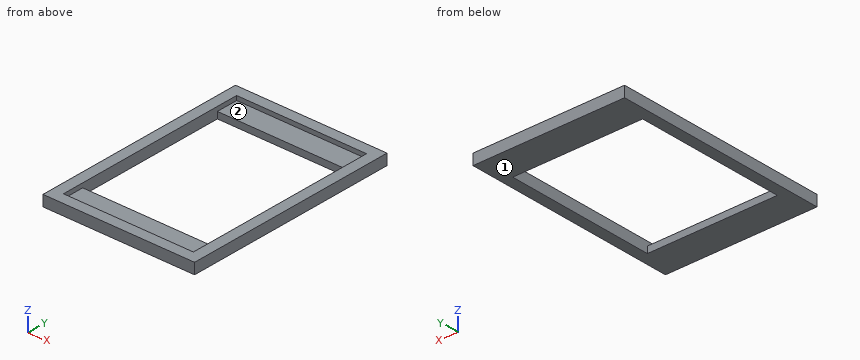
from build123d import *

# Parameters (mm, degrees)
SKETCH1_W           = 100
SKETCH1_H           = 70
BOSS_EXTRUDE1_DEPTH = 5
SKETCH2_W           = 60
SKETCH2_H           = 90
CUT_EXTRUDE1_DEPTH  = 62.23724357
SKETCH4_W           = 60
SKETCH4_H           = 3
BOSS_EXTRUDE2_DEPTH = 10
SKETCH5_W           = 60
SKETCH5_H           = 3
BOSS_EXTRUDE3_DEPTH = 10


with BuildPart() as part:
    # Sketch1 → Boss-Extrude1 (new body)
    with BuildSketch(Plane(origin=(0, 0, 0), x_dir=(0, 1, 0), z_dir=(0, 0, 1))):
        Rectangle(SKETCH1_W, SKETCH1_H)
    extrude(amount=BOSS_EXTRUDE1_DEPTH)

    # Sketch2 → Cut-Extrude1 (cut, through all)
    with BuildSketch(Plane.XY.offset(5)):
        Rectangle(SKETCH2_W, SKETCH2_H)
    extrude(amount=-CUT_EXTRUDE1_DEPTH, mode=Mode.SUBTRACT)

    # Sketch4 → Boss-Extrude2 (add)
    with BuildSketch(Plane.XZ.offset(-45)):
        with Locations((0, 1.5)):
            Rectangle(SKETCH4_W, SKETCH4_H)
    extrude(amount=BOSS_EXTRUDE2_DEPTH)

    # Sketch5 → Boss-Extrude3 (add)
    with BuildSketch(Plane(origin=(-45, -45, 0), x_dir=(1, 0, 0), z_dir=(0, 1, 0))):
        with Locations((45, -1.5)):
            Rectangle(SKETCH5_W, SKETCH5_H)
    extrude(amount=BOSS_EXTRUDE3_DEPTH)


solid = part.part
For this review, take the finished solid that the model builds, in its own axes (mm). Face numbers are marked on the shaded views. Round coordinates to 2 decimals unless told otherwise and drop trailing zeros. Loops run counter-clockwise (first coordinate to the right, second up) from the corner with the lowest first, then second, coordinate; pieces in that order, holes last. Notation, with made-up numbers: (77, 88.25) - (85, 88.25) arc R10 cw to (85, 101.25) - close; hole circle Ø8 at (55, 60.25). An arc over 180 degrees is marked (long way). Use one line per item in the form item = value.
1) Wall thickness on probe 1 along Y at (x, z) = (-4.5, 4.2); probe 2 along X at (y, z) = (12.5, 3.4); probe 3 along Y at (x, z) = (-16.5, 1.8): over which ranges is each line inside the solid? List them lowest first.
Solutions:
probe_1 = -50 to -45, 45 to 50
probe_2 = -35 to -30, 30 to 35
probe_3 = -50 to -35, 35 to 50
2) We need section B-B on z = 3.85. Write out the cut boundary in (x, y).
Solutions:
outline = (-35, -50) - (35, -50) - (35, 50) - (-35, 50) - close; hole (-30, -45) - (30, -45) - (30, 45) - (-30, 45) - close
3) We need section D-D on y = -42.5. Write out the cut boundary in (x, z), then the cut area to 3 significant figures.
Solutions:
outline = (-35, 0) - (35, 0) - (35, 5) - (30, 5) - (30, 3) - (-30, 3) - (-30, 5) - (-35, 5) - close
area = 230 mm2
4) We need section A-A on x = 15. Write out the cut boundary in (y, z), then the cut area to 3 significant figures.
Solutions:
outline = (-50, 0) - (-35, 0) - (-35, 3) - (-45, 3) - (-45, 5) - (-50, 5) - close; (35, 0) - (50, 0) - (50, 5) - (45, 5) - (45, 3) - (35, 3) - close
area = 110 mm2
5) Mouldability with a two-part tool opening along Y and no side actions: class the marked faces 1 and 2 as pulls with the +Y half, pulls with the -Y half, needs draft (parallel to the pull), parting line crosses it, or undercut.
Solutions:
face_1 = needs draft
face_2 = undercut
6) We need section C-C on y = -13. Write out the cut boundary in (x, z), then the cut area to 3 significant figures.
Solutions:
outline = (-35, 0) - (-30, 0) - (-30, 5) - (-35, 5) - close; (30, 0) - (35, 0) - (35, 5) - (30, 5) - close
area = 50.0 mm2
7) Clearance check with a flat-ended pin moving along its axis: P1, Ø5, axis at x = -7, y = -42, coming from the +Z side. State where the tip first meets the part, or that it passes through.
Solutions:
P1 = 3
